Can you work these out from the model? Positions are in its coordinate system, mm. A direction names the side the tool comes from. Coordinates: 2 decimals unless noted, no trailing zeros. Order: outer loops, then holes, each group sorted by start corner. A loop starts at its lowest first (then second) coordinate and runs counter-clockwise, first axis right, second up. Notation, with made-up numbers: (59.5, -24) - (82.5, -24) arc R22 cw to (82.5, -18) - close; hole circle Ø1 at (69.25, 84). An arc over 180 degrees is marked (long way). Return JSON: item names as keys, results as strings. Group by question number.
1) Which directions (+Z, -Z, +X, -X, +Y, -Y) give clear straight access to the entire face, cutting with the end or side of a thin tool? Please do faces 1 (the face through (0.54, 1.48, -2.44)), 2 (the face through (0.54, -1.99, -2.44)), 3 (the face through (0, 3, 0)).
2) Imagine slicing it at B-B (z = 0). Write out the boundary of the cut face in (x, y), and give its area (3 significant figures).
3) If I drill on line 1 along Y through (x, z) = (1, 5); line 2 along X through (y, z) = (-0.9, -11.5); line 3 along X through (y, z) = (-0.65, -1.5), over which ranges is the centre line in solid material (lowest first)?
4) For pin 1 Ø1.5 at (x, z) = (-10.5, -13.5) entering from -Y; pin 2 Ø1.5 at (x, y) = (4, 1) entering from -Z; pin 3 Ø5 at (x, z) = (-9, -2) entering from +Y, each with a flat end and sliding along its axis, tell me the tip position at first contact or that it passes through.
5) Imagine slicing it at A-A (x = 0). Write out the boundary of the cut face in (y, z), and give its area (3 significant figures).
6) Imagine slicing it at C-C (y = 2.3). Write out the boundary of the cut face in (x, z), and give its area (3 significant figures).
7) Imagine slicing it at D-D (z = 14). Write out the boundary of the cut face in (x, y), and give its area (3 significant figures).
```python
from build123d import *

# Parameters (mm, degrees)
F0_W     = 1
F0_H     = 17.5
F2_R     = 2.5
F3_DEPTH = 3
F4_DEPTH = 6


with BuildPart() as f1:
    # F0 (on Right) → F1 (revolve)
    with BuildSketch(Plane.YZ):
        with Locations((-0.5, 8.75)):
            Rectangle(F0_W, F0_H)
    revolve(axis=Axis((0, -0.5, 0), (0, 1, 0)))

    # F2 (on face) → F3 (join)
    with BuildSketch(Plane(origin=(0, 0, 0), x_dir=(-1, 0, 0), z_dir=(0, 1, 0))):
        Circle(F2_R)
    extrude(amount=F3_DEPTH)

    # F4 (add): a face of the model
    f4_faces = [f1.faces().sort_by_distance(p)[0] for p in [
        (0, 3, 0),
    ]]
    extrude(f4_faces, amount=-F4_DEPTH)


solid = f1.part
```
Calculated:
{
 "1": {"face 1": "+Y", "face 2": "-Y", "face 3": "+Z, -Z, +X, -X, +Y"},
 "2": {"outline": "(-17.5, -1) - (-2.5, -1) - (-2.5, -3) - (2.5, -3) - (2.5, -1) - (17.5, -1) - (17.5, 0) - (2.5, 0) - (2.5, 3) - (-2.5, 3) - (-2.5, 0) - (-17.5, 0) - close", "area": "60.0 mm2"},
 "3": {"line 1": "-1 to 0", "line 2": "-13.19 to 13.19", "line 3": "-17.44 to 17.44"},
 "4": {"pin 1": "y = -1", "pin 2": "through", "pin 3": "y = 0"},
 "5": {"outline": "(-3, -2.5) - (-1, -2.5) - (-1, -17.5) - (0, -17.5) - (0, -2.5) - (3, -2.5) - (3, 2.5) - (0, 2.5) - (0, 17.5) - (-1, 17.5) - (-1, 2.5) - (-3, 2.5) - close", "area": "60.0 mm2"},
 "6": {"outline": "circle Ø5 at (0, 0)", "area": "19.6 mm2"},
 "7": {"outline": "(-10.5, -1) - (10.5, -1) - (10.5, 0) - (-10.5, 0) - close", "area": "21.0 mm2"}
}
